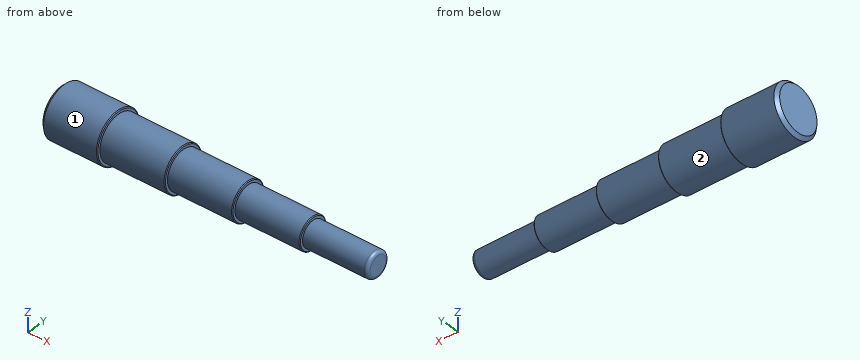
from build123d import *

# Parameters (mm, degrees)
F2_SIZE = 2
F3_SIZE = 0.5
F4_R    = 2


with BuildPart() as f1:
    # F0 (on Front) → F1 (revolve)
    with BuildSketch(Plane.XZ):
        Polygon((-200, 0), (0, 0), (0, 8), (-41, 8), (-41, 10), (-82, 10), (-82, 12), (-123, 12), (-123, 14), (-164, 14), (-164, 16), (-200, 16), align=None)
    revolve(axis=Axis((-100, 0, 0), (-1, 0, 0)))

    # F2
    f2_edges = [f1.edges().sort_by_distance(p)[0] for p in [
        (-200, 0, -16),
    ]]
    chamfer(f2_edges, length=F2_SIZE)

    # F3
    f3_edges = [f1.edges().sort_by_distance(p)[0] for p in [
        (-164, 0, -16),
        (-123, 0, -14),
        (-82, 0, -12),
        (-41, 0, -10),
    ]]
    chamfer(f3_edges, length=F3_SIZE)

    # F4
    f4_edges = [f1.edges().sort_by_distance(p)[0] for p in [
        (0, 0, -8),
    ]]
    fillet(f4_edges, radius=F4_R)


solid = f1.part
The listing builds one solid part. Answer for the finished solid, in the listing's coordinates (mm). Face numbers are marked on the shaded views. A direction names the side the tool comes from. Give positions to 0.01 mm unless a question says otherwise; leave off trailing zeros. Loops run counter-clockwise (first coordinate to the right, second up) from the corner with the lowest first, then second, coordinate; pieces in that order, holes last. Notation, with made-up numbers: (-37.5, -32.5) - (-27.5, -32.5) arc R21 cw to (-27.5, -5.5) - close; hole circle Ø3 at (-24, 73). An arc over 180 degrees is marked (long way). Write each question's results on one line, items separated by ' | '.
1. Flat-ended cylindrical pins translate along their axes: P1, Ø3, axis at x = -165.5, y = 10.5, coming from the -Z side; P2, Ø1, axis at x = -157.5, y = 8, coming from the +Z side; P3, Ø1.5, axis at x = -131.5, y = -7, coming from the -Z side; P4, Ø9.5, axis at y = -0.5, z = 3, coming from the +X side. Find the tip coordinate at first contact, or state that the pin passes through.
Resolved:
P1: stops at z = -13.23 | P2: stops at z = 11.82 | P3: stops at z = -12.53 | P4: stops at x = 0
2. Consider probe 1 along Y at (x, z) = (-109, 3.5); probe 2 along X at (y, z) = (-3, 5.5); probe 3 along X at (y, z) = (8, 7.5). Determine where each line is inside the solid, lowest interval first. Write a range as from..to.
Resolved:
probe 1: y = -11.48..11.48 | probe 2: x = -200..-0.02 | probe 3: x = -200..-82
3. Find section D-D, the plane x = -91.5. Write down the section's boundary in (y, z), then the cut area to 3 significant figures.
Resolved:
outline: circle Ø24 at (0, 0) | area: 452 mm^2
4. Which of the six approach directions +Z, -Z, +X, -X, +Y, -Y give full straight-line access (tool end or side, diameter ignored) to the marked faces 1 and 2?
Resolved:
face 1: +X, -X | face 2: +X
5. Find section C-C, the plane x = -31.5. Write down the section's boundary in (y, z), then the cut area to 3 significant figures.
Resolved:
outline: circle Ø16 at (0, 0) | area: 201 mm^2
